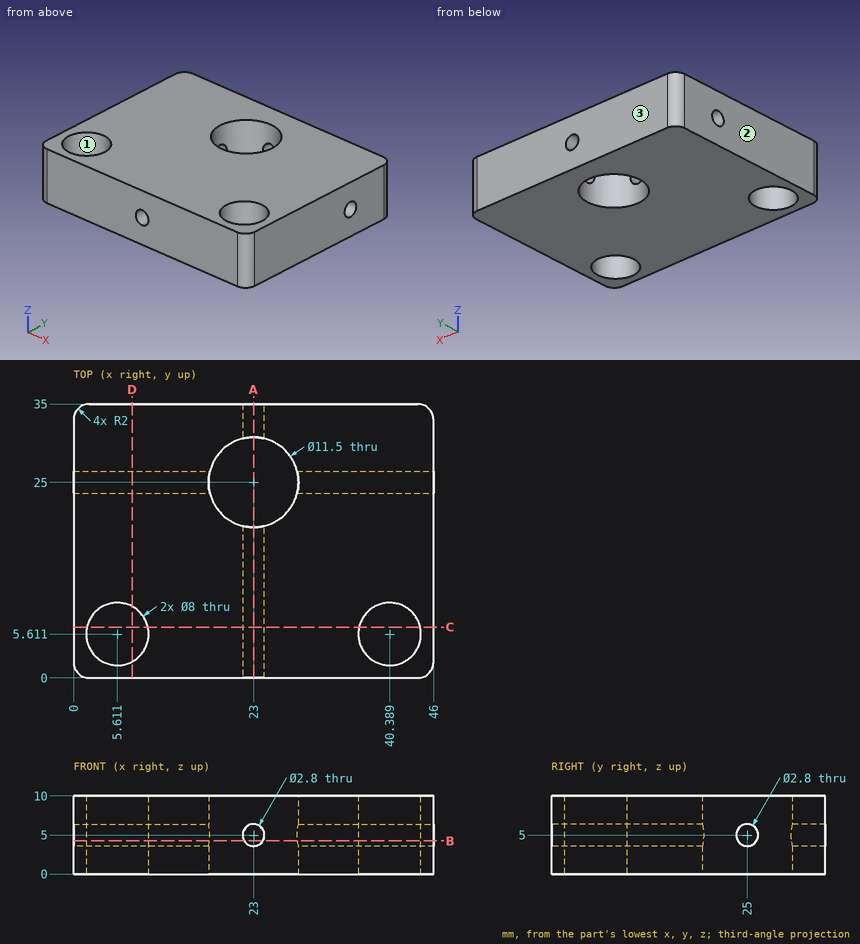
Check sheet for the drawn part. Datum: minimum x, y, z corner. Units: mm. Round coordinates to 2 decimals unless told otherwise and drop trailing zeros. Order: outer loops, then holes, each group sorted by start corner. A loop starts at its lowest first (then second) coordinate and runs counter-clockwise, first axis right, second up. Notation, with made-up numbers: (40, -11) -> (85, -11) arc R25 ccw to (85, 1) -> close; hole circle Ø3 at (85, 46.5). An arc over 180 degrees is marked (long way). Put each result on its own line as item: value. Start each with the question number.
(1) Section check C-C (y = 6.5). Enter the section's corners in (x, z).
(2) Section check B-B (z = 4.25). Enter the section's corners in (x, y).
(3) Draft check along Y on the marked faces 1, 2 and 3. Enter one of: +Y half, -Y half, draft (parallel to the pull), parting line (faces both ways), or undercut.
(4) Material ranges on line 1 along Y through (x, z) = (40.5, 5); line 2 along Y through (x, z) = (6, 4); line 3 along Y through (x, z) = (35.75, 5), recorded low to high.
(5) Section check A-A (x = 23). Enter the section's corners in (y, z), then the cut area to 3 significant figures.
(6) Section check D-D (x = 7.5). Enter the section's corners in (y, z) (1 decimal), then the cut area to 3 significant figures.
Completed:
1. outline: (0, 0) -> (1.71, 0) -> (1.71, 10) -> (0, 10) -> close; (9.51, 0) -> (36.49, 0) -> (36.49, 10) -> (9.51, 10) -> close; (44.29, 0) -> (46, 0) -> (46, 10) -> (44.29, 10) -> close; hole circle Ø2.8 at (23, 5)
2. outline: (0, 2) arc R2 ccw to (2, 0) -> (21.82, 0) -> (21.82, 19.37) arc R5.75 cw to (17.37, 23.82) -> (0, 23.82) -> close; (0, 26.18) -> (17.37, 26.18) arc R5.75 cw to (21.82, 30.63) -> (21.82, 35) -> (2, 35) arc R2 ccw to (0, 33) -> close; (24.18, 0) -> (44, 0) arc R2 ccw to (46, 2) -> (46, 23.82) -> (28.63, 23.82) arc R5.75 cw to (24.18, 19.37) -> close; (24.18, 30.63) arc R5.75 cw to (28.63, 26.18) -> (46, 26.18) -> (46, 33) arc R2 ccw to (44, 35) -> (24.18, 35) -> close; hole circle Ø8 at (5.61, 5.61); hole circle Ø8 at (40.39, 5.61)
3. face 1: undercut
3. face 2: draft
3. face 3: +Y half
4. line 1: y = 0 to 1.61, 9.61 to 23.6, 26.4 to 35
4. line 2: y = 0 to 1.63, 9.59 to 24.02, 25.98 to 35
4. line 3: y = 0 to 23.6, 26.4 to 35
5. outline: (0, 0) -> (19.25, 0) -> (19.25, 3.6) -> (0, 3.6) -> close; (0, 6.4) -> (19.25, 6.4) -> (19.25, 10) -> (0, 10) -> close; (30.75, 0) -> (35, 0) -> (35, 3.6) -> (30.75, 3.6) -> close; (30.75, 6.4) -> (35, 6.4) -> (35, 10) -> (30.75, 10) -> close
5. area: 169 mm2
6. outline: (0, 0) -> (2.1, 0) -> (2.1, 10) -> (0, 10) -> close; (9.1, 0) -> (35, 0) -> (35, 10) -> (9.1, 10) -> close; hole circle Ø2.8 at (25, 5)
6. area: 273 mm2
